For this review, take the finished solid that the model builds, in its own axes (mm). Face numbers are marked on the shaded views. A direction names the side the tool comes from. Coordinates: 2 decimals unless noted, no trailing zeros. Write each loop counter-clockwise with the first axis right and the second up, starting at its lowest first coordinate (ties: lowest second). Pieces come first, ordered by that corner, then holes.
```python
from build123d import *

# Parameters (mm, degrees)
SKETCH1_W           = 111
SKETCH1_H           = 60
BOSS_EXTRUDE1_DEPTH = 43.5
SKETCH2_W           = 101
SKETCH2_H           = 50
CUT_EXTRUDE1_DEPTH  = 18
CUT_EXTRUDE3_DEPTH  = 23
CUT_EXTRUDE5_START  = -2
SKETCH5_W           = 68.5
SKETCH5_H           = 50
CUT_EXTRUDE5_DEPTH  = 18.5
SKETCH6_W           = 37.5
SKETCH6_H           = 60
CUT_EXTRUDE6_DEPTH  = 2.5
SKETCH7_R           = 1
CUT_EXTRUDE7_DEPTH  = 4
SKETCH8_R           = 1
CUT_EXTRUDE8_DEPTH  = 4
SKETCH9_W           = 19
SKETCH9_H           = 13
CUT_EXTRUDE9_DEPTH  = 10
SKETCH12_W          = 30
SKETCH12_H          = 3
CUT_EXTRUDE12_DEPTH = 32.5
FILLET2_R           = 2.5
FILLET3_R           = 2.5
FILLET4_R           = 2.5
FILLET5_R           = 2.5
FILLET6_R           = 2.5
SKETCH13_W          = 27.5
SKETCH13_H          = 56
CUT_EXTRUDE13_DEPTH = 17
SKETCH14_W          = 15
SKETCH14_H          = 10
CUT_EXTRUDE14_DEPTH = 25
FILLET7_R           = 1.5
FILLET8_R           = 1.5
FILLET9_R           = 1.5
FILLET10_R          = 1.5
FILLET11_R          = 2.5
FILLET12_R          = 1.5
SKETCH15_W          = 22.107435613
SKETCH15_H          = 4.839639835
CUT_EXTRUDE15_DEPTH = 10
SKETCH16_W          = 15
SKETCH16_H          = 2.5
CUT_EXTRUDE16_DEPTH = 61


with BuildPart() as part:
    # Sketch1 → Boss-Extrude1 (new body)
    with BuildSketch(Plane(origin=(0, 0, 0), x_dir=(1, 0, 0), z_dir=(0, 1, 0))):
        with Locations((55.5, 30)):
            Rectangle(SKETCH1_W, SKETCH1_H)
    extrude(amount=BOSS_EXTRUDE1_DEPTH)

    # Sketch2 → Cut-Extrude1 (cut)
    with BuildSketch(Plane(origin=(0, 43.5, 0), x_dir=(1, 0, 0), z_dir=(0, 1, 0))):
        with Locations((55.5, 30)):
            Rectangle(SKETCH2_W, SKETCH2_H)
    extrude(amount=-CUT_EXTRUDE1_DEPTH, mode=Mode.SUBTRACT)

    # Sketch3 → Cut-Extrude3 (cut)
    with BuildSketch(Plane(origin=(0, 43.5, 0), x_dir=(1, 0, 0), z_dir=(0, 1, 0))):
        Polygon((5, 45), (15, 45), (15, 55), (96, 55), (96, 45), (106, 45), (106, 15), (96, 15), (96, 5), (15, 5), (15, 15), (5, 15), align=None)
    extrude(amount=-CUT_EXTRUDE3_DEPTH, mode=Mode.SUBTRACT)

    # Sketch5 → Cut-Extrude5 (cut)
    with BuildSketch(Plane.XZ.offset(CUT_EXTRUDE5_START)):
        with Locations((71.75, -30)):
            Rectangle(SKETCH5_W, SKETCH5_H)
    extrude(amount=-CUT_EXTRUDE5_DEPTH, mode=Mode.SUBTRACT)

    # Sketch6 → Cut-Extrude6 (cut)
    with BuildSketch(Plane.XZ):
        with Locations((18.75, -30)):
            Rectangle(SKETCH6_W, SKETCH6_H)
    extrude(amount=-CUT_EXTRUDE6_DEPTH, mode=Mode.SUBTRACT)

    # Sketch7 → Cut-Extrude7 (cut)
    with BuildSketch(Plane(origin=(0, 2.5, 0), x_dir=(-1, 0, 0), z_dir=(0, -1, 0))):
        with Locations((-2.5, 57.5)):
            Circle(SKETCH7_R)
        with Locations((-35, 57.5)):
            Circle(SKETCH7_R)
        with Locations((-35, 2.5)):
            Circle(SKETCH7_R)
        with Locations((-2.5, 2.5)):
            Circle(SKETCH7_R)
    extrude(amount=-CUT_EXTRUDE7_DEPTH, mode=Mode.SUBTRACT)

    # Sketch8 → Cut-Extrude8 (cut)
    with BuildSketch(Plane(origin=(0, 43.5, 0), x_dir=(1, 0, 0), z_dir=(0, 1, 0))):
        with Locations((2.5, 57.5)):
            Circle(SKETCH8_R)
        with Locations((108.5, 57.5)):
            Circle(SKETCH8_R)
        with Locations((108.5, 2.360383006)):
            Circle(SKETCH8_R)
        with Locations((2.5, 2.5)):
            Circle(SKETCH8_R)
    extrude(amount=-CUT_EXTRUDE8_DEPTH, mode=Mode.SUBTRACT)

    # Sketch9 → Cut-Extrude9 (cut)
    with BuildSketch(Plane.XY):
        with Locations((82, 9.5)):
            Rectangle(SKETCH9_W, SKETCH9_H)
    extrude(amount=-CUT_EXTRUDE9_DEPTH, mode=Mode.SUBTRACT)

    # Sketch12 → Cut-Extrude12 (cut)
    with BuildSketch(Plane(origin=(0, 43.5, 0), x_dir=(1, 0, 0), z_dir=(0, 1, 0))):
        with Locations((56, 56.5)):
            Rectangle(SKETCH12_W, SKETCH12_H)
    extrude(amount=-CUT_EXTRUDE12_DEPTH, mode=Mode.SUBTRACT)

    # Fillet2
    fillet2_edges = [part.edges().sort_by_distance(p)[0] for p in [
        (0, 23, 0),
    ]]
    fillet(fillet2_edges, radius=FILLET2_R)

    # Fillet3
    fillet3_edges = [part.edges().sort_by_distance(p)[0] for p in [
        (111, 21.75, 0),
    ]]
    fillet(fillet3_edges, radius=FILLET3_R)

    # Fillet4
    fillet4_edges = [part.edges().sort_by_distance(p)[0] for p in [
        (0, 23, -60),
    ]]
    fillet(fillet4_edges, radius=FILLET4_R)

    # Fillet5
    fillet5_edges = [part.edges().sort_by_distance(p)[0] for p in [
        (111, 21.75, -60),
    ]]
    fillet(fillet5_edges, radius=FILLET5_R)

    # Fillet6
    fillet6_edges = [part.edges().sort_by_distance(p)[0] for p in [
        (73, 0, -60),
        (110.267766953, 0, -59.267766953),
        (111, 0, -30),
        (110.267766953, 0, -0.732233047),
        (73, 0, 0),
    ]]
    fillet(fillet6_edges, radius=FILLET6_R)

    # Sketch13 → Cut-Extrude13 (cut)
    with BuildSketch(Plane.XZ.offset(-2.5)):
        with Locations((18.75, -30)):
            Rectangle(SKETCH13_W, SKETCH13_H)
    extrude(amount=-CUT_EXTRUDE13_DEPTH, mode=Mode.SUBTRACT)

    # Sketch14 → Cut-Extrude14 (cut, through all)
    with BuildSketch(Plane.XZ.offset(-19.5)):
        with Locations((24.5, -11.134142308)):
            Rectangle(SKETCH14_W, SKETCH14_H)
    extrude(amount=-CUT_EXTRUDE14_DEPTH, mode=Mode.SUBTRACT)

    # Fillet7
    fillet7_edges = [part.edges().sort_by_distance(p)[0] for p in [
        (32.5, 11, -2),
    ]]
    fillet(fillet7_edges, radius=FILLET7_R)

    # Fillet8
    fillet8_edges = [part.edges().sort_by_distance(p)[0] for p in [
        (5, 11, -2),
    ]]
    fillet(fillet8_edges, radius=FILLET8_R)

    # Fillet9
    fillet9_edges = [part.edges().sort_by_distance(p)[0] for p in [
        (32.5, 11, -58),
    ]]
    fillet(fillet9_edges, radius=FILLET9_R)

    # Fillet10
    fillet10_edges = [part.edges().sort_by_distance(p)[0] for p in [
        (5, 11, -58),
    ]]
    fillet(fillet10_edges, radius=FILLET10_R)

    # Fillet11
    fillet11_edges = [part.edges().sort_by_distance(p)[0] for p in [
        (37.5, 20.5, -30),
    ]]
    fillet(fillet11_edges, radius=FILLET11_R)

    # Fillet12
    fillet12_edges = [part.edges().sort_by_distance(p)[0] for p in [
        (71, 27.25, -55),
        (41, 27.25, -55),
    ]]
    fillet(fillet12_edges, radius=FILLET12_R)

    # Sketch15 → Cut-Extrude15 (cut)
    with BuildSketch(Plane(origin=(37.5, 0, 0), x_dir=(0, 0, -1), z_dir=(1, 0, 0))):
        with Locations((18.663805006, 13.487875839)):
            Rectangle(SKETCH15_W, SKETCH15_H)
    extrude(amount=-CUT_EXTRUDE15_DEPTH, mode=Mode.SUBTRACT)

    # Sketch16 → Cut-Extrude16 (cut, through all)
    with BuildSketch(Plane.XY):
        with Locations((55.5, 2.25)):
            Rectangle(SKETCH16_W, SKETCH16_H)
    extrude(amount=-CUT_EXTRUDE16_DEPTH, mode=Mode.SUBTRACT)


solid = part.part
```
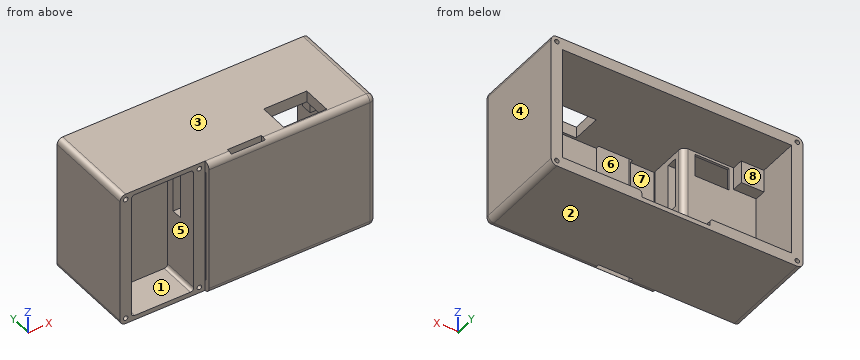
1) Clearance check with flat-ended pins moving along their axes: P1, Ø5, axis at x = 71.5, z = -47.5, coming from the +Y side; P2, Ø2, axis at y = 1, z = -33.5, coming from the -X side; P3, Ø11, axis at x = 14, z = -37, coming from the -Y side. State where each tip first meets the part, or that it passes through.
2) Consider section A-A (z = -51.5). Give the boundary of the cut face in (x, y).
3) Tool access review of the marked faces 5, 6, 7 and 8: name each direction out of +Z, -Z, +X, -X, +Y, -Y from which nothing blocks a thin tool from reaching the whole face with its end or side.
4) For L1, parallel to X at y = 7, z = -45; L2, parallel to Z at x = 35, y = 5.6; L3, parallel to X at y = 41.05, z = -57.5, list the stretches that pass through material, from the lowest coordinate up.
5) Consider section B-B (y = 32). Give the boundary of the cut face in (x, z).
6) Consider section C-C (z = -22). Give the boundary of the cut face in (x, y).
7) The part is to be moulded in two halves that separate along Z. For the marked faces 1, 2, 3 and 4, say which applies: pulls with the +Z half, pulls with the -Z half, needs draft (parallel to the pull), parting line crosses it, or undercut.
Results:
1. P1: stops at y = 2
1. P2: stops at x = 37.5
1. P3: stops at y = 19.5
2. outline: (0, 2.5) - (5, 2.5) - (5, 19.5) - (32.5, 19.5) - (32.5, 2.5) - (37.5, 2.5) - (37.5, 18) arc R2.5 ccw to (35, 20.5) - (15, 20.5) - (15, 25.5) - (5, 25.5) - (5, 43.5) - (0, 43.5) - close; (37.5, 0) - (108.5, 0) arc R2.5 ccw to (111, 2.5) - (111, 43.5) - (106, 43.5) - (106, 25.5) - (96, 25.5) - (96, 20.5) - (106, 20.5) - (106, 2) - (63, 2) - (63, 1) - (48, 1) - (48, 2) - (37.5, 2) - close
3. face 5: -Y
3. face 6: +Z, -Z
3. face 7: -X, +Y
3. face 8: +Y
4. L1: x = 0 to 5, 32.5 to 37.5, 106 to 111
4. L2: z = -60 to -58.5, -56.5 to -3.5, -1.5 to 0
4. L3: x = 0 to 1.5, 3.5 to 41, 71 to 107.5, 109.5 to 111
5. outline: (0, -57.5) arc R2.5 ccw to (2.5, -60) - (108.5, -60) arc R2.5 ccw to (111, -57.5) - (111, -2.5) arc R2.5 ccw to (108.5, 0) - (2.5, 0) arc R2.5 ccw to (0, -2.5) - close; hole (5, -55) - (39.5, -55) arc R1.5 cw to (41, -56.5) - (41, -58) - (71, -58) - (71, -56.5) arc R1.5 cw to (72.5, -55) - (106, -55) - (106, -5) - (5, -5) - close
6. outline: (0, 2.5) - (5, 2.5) - (5, 19.5) - (32.5, 19.5) - (32.5, 15.91) - (37.5, 15.91) - (37.5, 18) arc R2.5 ccw to (35, 20.5) - (5, 20.5) - (5, 43.5) - (0, 43.5) - close; (32.5, 2.5) - (37.5, 2.5) - (37.5, 11.07) - (32.5, 11.07) - close; (37.5, 0) - (108.5, 0) arc R2.5 ccw to (111, 2.5) - (111, 43.5) - (106, 43.5) - (106, 2) - (63, 2) - (63, 1) - (48, 1) - (48, 2) - (37.5, 2) - close
7. face 1: undercut
7. face 2: pulls with the -Z half
7. face 3: pulls with the +Z half
7. face 4: needs draft
